from build123d import *

# Parameters (mm, degrees)
F0_R     = 22.225
F0_R_2   = 2.15265
F0_R_3   = 3.96875
F1_DEPTH = 32.593001
F2_R     = 3.96875
F3_DEPTH = 6.35


with BuildPart() as f1:
    # F0 (on Top) → F1 (new body)
    with BuildSketch(Plane.XY):
        Circle(F0_R)
        with Locations((-11.786586, -11.786586)):
            Circle(F0_R_2, mode=Mode.SUBTRACT)
        with Locations((11.786586, -11.786586)):
            Circle(F0_R_2, mode=Mode.SUBTRACT)
        with Locations((0, -9.525)):
            Circle(F0_R_2, mode=Mode.SUBTRACT)
        with Locations((-11.786586, 11.786586)):
            Circle(F0_R_2, mode=Mode.SUBTRACT)
        Circle(F0_R_3, mode=Mode.SUBTRACT)
        with Locations((0, 9.525)):
            Circle(F0_R_2, mode=Mode.SUBTRACT)
        with Locations((11.786586, 11.786586)):
            Circle(F0_R_2, mode=Mode.SUBTRACT)
    extrude(amount=F1_DEPTH)

    # F2 (on face) → F3 (cut)
    with BuildSketch(Plane.XY.offset(32.593001)):
        with Locations((-11.786586, 11.786586)):
            Circle(F2_R)
        with Locations((11.786586, -11.786586)):
            Circle(F2_R)
    extrude(amount=-F3_DEPTH, mode=Mode.SUBTRACT)


solid = f1.part
The model under review builds one solid part; all positions refer to its coordinate system, in mm. A direction names the side the tool comes from. Round coordinates to 2 decimals unless told otherwise and drop trailing zeros. Write each loop counter-clockwise with the first axis right and the second up, starting at its lowest first coordinate (ties: lowest second). Pieces come first, ordered by that corner, then holes. Notation, with made-up numbers: M 77.25,-16 L 103.25,-16 A31 ccw 103.25,8 Z; hole C -21,-37.75 d8. An arc over 180 degrees is marked long. Use a Markdown table: item, result. Add a question column.
Q1. We need section B-B, the plane y = 0. State the section outline as (x, z) points (3 decimals), plus the area to 3 significant figures.
Q2. We need section A-A, the plane x = 0. State the section outline as (y, z) points (3 decimals).
Q3. We need section C-C, the plane z = 30.5. Count the separate pieces of the cut face and the enclosed holes in it, plus the area to 3 significant figures.
Q4. To check wall thickness, follow line 1 (Y direction, x = 0, z = 8) (3 decimals); line 2 (Y direction, x = 11, z = 13); line 3 (X direction, y = -13, z = 21.5). State the ranges of each line that lie inside material, in increasing order.
Q5. Insertion check: pin 1 (6.5 mm diameter, centred on x = 0, y = 0, fed in from -Z); pin 2 (6 mm diameter, centred on x = 7, z = 3.5, fed in from -Y); pin 3 (5 mm diameter, centred on y = 5, z = 19, fed in from +X); pin 4 (10 mm diameter, centred on y = -11, z = 27, fed in from +X). Each pin has a flat end and moves straight along its axis. Give the tip position at first contact, or say it passes through.
Q6. Machinability: for faces 1 (the face through (8.637, -14.202, 29.462)), 2 (the face through (10.08, -13.1, 12.94)), which of the approach directions +Z, -Z, +X, -X, +Y, -Y give a long, thin tool a straight path to every point of the face, cutting with its end or side? Answer none if there is none.
Findings below:
| question | item | result |
|---|---|---|
| 1 | outline | M -22.225,0 L -3.969,0 L -3.969,32.593 L -22.225,32.593 Z; M 3.969,0 L 22.225,0 L 22.225,32.593 L 3.969,32.593 Z |
| 1 | area | 1,190 mm² |
| 2 | outline | M -22.225,0 L -11.678,0 L -11.678,32.593 L -22.225,32.593 Z; M -7.372,0 L -3.969,0 L -3.969,32.593 L -7.372,32.593 Z; M 3.969,0 L 7.372,0 L 7.372,32.593 L 3.969,32.593 Z; M 11.678,0 L 22.225,0 L 22.225,32.593 L 11.678,32.593 Z |
| 3 | separate pieces | 1 |
| 3 | enclosed holes | 7 |
| 3 | area | 1,350 mm² |
| 4 | line 1 | y = -22.225 to -11.678, -7.372 to -3.969, 3.969 to 7.372, 11.678 to 22.225 |
| 4 | line 2 | y = -19.31 to -13.79, -9.78 to 9.78, 13.79 to 19.31 |
| 4 | line 3 | x = -18.03 to -13.56, -10.01 to 10.01, 13.56 to 18.03 |
| 5 | pin 1 | passes through |
| 5 | pin 2 | stops at y = -21.86 |
| 5 | pin 3 | stops at x = 22.08 |
| 5 | pin 4 | stops at x = 21.4 |
| 6 | face 1 | +Z |
| 6 | face 2 | +Z, -Z |
